from build123d import *

# Parameters (mm, degrees)
SKETCH_1_R      = 31.73899895
SKETCH_1_R_2    = 15.869499475
SKETCH_1_R_3    = 1.5
EXTRUDE_2_DEPTH = 2
EXTRUDE_3_DEPTH = 3
FILLET_1_R      = 1
FILLET_2_R      = 1
FILLET_3_R      = 1
FILLET_4_R      = 1
FILLET_5_R      = 1
FILLET_6_R      = 1
FILLET_7_R      = 1
FILLET_8_R      = 1


with BuildPart() as part:
    # 草图1 → 凸台-拉伸2 (new body)
    with BuildSketch(Plane.XY):
        Circle(SKETCH_1_R)
        Circle(SKETCH_1_R_2, mode=Mode.SUBTRACT)
        with Locations((-17, 17)):
            Circle(SKETCH_1_R_3, mode=Mode.SUBTRACT)
        with Locations((17, 17)):
            Circle(SKETCH_1_R_3, mode=Mode.SUBTRACT)
        with Locations((17, -17)):
            Circle(SKETCH_1_R_3, mode=Mode.SUBTRACT)
        with Locations((-17, -17)):
            Circle(SKETCH_1_R_3, mode=Mode.SUBTRACT)
        with Locations((-19.798989873, 19.798989873)):
            Circle(SKETCH_1_R_3, mode=Mode.SUBTRACT)
        with Locations((0, 28)):
            Circle(SKETCH_1_R_3, mode=Mode.SUBTRACT)
        with Locations((19.798989873, 19.798989873)):
            Circle(SKETCH_1_R_3, mode=Mode.SUBTRACT)
        with Locations((28, 0)):
            Circle(SKETCH_1_R_3, mode=Mode.SUBTRACT)
        with Locations((19.798989873, -19.798989873)):
            Circle(SKETCH_1_R_3, mode=Mode.SUBTRACT)
        with Locations((0, -28)):
            Circle(SKETCH_1_R_3, mode=Mode.SUBTRACT)
        with Locations((-19.798989873, -19.798989873)):
            Circle(SKETCH_1_R_3, mode=Mode.SUBTRACT)
        with Locations((-28, 0)):
            Circle(SKETCH_1_R_3, mode=Mode.SUBTRACT)
    extrude(amount=EXTRUDE_2_DEPTH)

    # 草图2 → 凸台-拉伸3 (add)
    with BuildSketch(Plane.XY.offset(2)):
        with BuildLine():
            Line((11.25, 23.25), (-11.25, 23.25))
            Line((-11.25, 23.25), (-11.25, 21.25))
            Line((-11.25, 21.25), (-4.584929155, 21.25))
            ThreePointArc((-4.584929155, 21.25), (0, 21.73899895), (4.584929155, 21.25))
            Line((4.584929155, 21.25), (11.25, 21.25))
            Line((11.25, 21.25), (11.25, 23.25))
        make_face()
        with BuildLine():
            Line((-23.25, 11.25), (-23.25, -11.25))
            Line((-23.25, -11.25), (-21.25, -11.25))
            Line((-21.25, -11.25), (-21.25, -4.584929155))
            ThreePointArc((-21.25, -4.584929155), (-21.73899895, 0), (-21.25, 4.584929155))
            Line((-21.25, 4.584929155), (-21.25, 11.25))
            Line((-21.25, 11.25), (-23.25, 11.25))
        make_face()
        with BuildLine():
            Line((21.25, -11.25), (23.25, -11.25))
            Line((23.25, -11.25), (23.25, 11.25))
            Line((23.25, 11.25), (21.25, 11.25))
            Line((21.25, 11.25), (21.25, 4.584929155))
            ThreePointArc((21.25, 4.584929155), (21.616403529, 2.305466077), (21.73899895, 0))
            ThreePointArc((21.73899895, 0), (21.616403529, -2.305466077), (21.25, -4.584929155))
            Line((21.25, -4.584929155), (21.25, -11.25))
        make_face()
        with BuildLine():
            Line((-11.25, -21.25), (-11.25, -23.25))
            Line((-11.25, -23.25), (11.25, -23.25))
            Line((11.25, -23.25), (11.25, -21.25))
            Line((11.25, -21.25), (4.584929155, -21.25))
            ThreePointArc((4.584929155, -21.25), (0, -21.73899895), (-4.584929155, -21.25))
            Line((-4.584929155, -21.25), (-11.25, -21.25))
        make_face()
        with BuildLine():
            ThreePointArc((-21.25, 4.584929155), (-21.73899895, 0), (-21.25, -4.584929155))
            Line((-21.25, -4.584929155), (-21.25, 4.584929155))
        make_face()
        with BuildLine():
            ThreePointArc((4.584929155, 21.25), (0, 21.73899895), (-4.584929155, 21.25))
            Line((-4.584929155, 21.25), (4.584929155, 21.25))
        make_face()
        with BuildLine():
            Line((21.25, 4.584929155), (21.25, -4.584929155))
            ThreePointArc((21.25, -4.584929155), (21.616403529, -2.305466077), (21.73899895, 0))
            ThreePointArc((21.73899895, 0), (21.616403529, 2.305466077), (21.25, 4.584929155))
        make_face()
    extrude(amount=EXTRUDE_3_DEPTH)

    # 圆角1
    fillet_1_edges = [part.edges().sort_by_distance(p)[0] for p in [
        (-22.25, -11.25, 5),
    ]]
    fillet(fillet_1_edges, radius=FILLET_1_R)

    # 圆角2
    fillet_2_edges = [part.edges().sort_by_distance(p)[0] for p in [
        (-22.25, 11.25, 5),
    ]]
    fillet(fillet_2_edges, radius=FILLET_2_R)

    # 圆角3
    fillet_3_edges = [part.edges().sort_by_distance(p)[0] for p in [
        (-11.25, 22.25, 5),
    ]]
    fillet(fillet_3_edges, radius=FILLET_3_R)

    # 圆角4
    fillet_4_edges = [part.edges().sort_by_distance(p)[0] for p in [
        (11.25, 22.25, 5),
    ]]
    fillet(fillet_4_edges, radius=FILLET_4_R)

    # 圆角5
    fillet_5_edges = [part.edges().sort_by_distance(p)[0] for p in [
        (22.25, 11.25, 5),
    ]]
    fillet(fillet_5_edges, radius=FILLET_5_R)

    # 圆角6
    fillet_6_edges = [part.edges().sort_by_distance(p)[0] for p in [
        (22.25, -11.25, 5),
    ]]
    fillet(fillet_6_edges, radius=FILLET_6_R)

    # 圆角7
    fillet_7_edges = [part.edges().sort_by_distance(p)[0] for p in [
        (11.25, -22.25, 5),
    ]]
    fillet(fillet_7_edges, radius=FILLET_7_R)

    # 圆角8
    fillet_8_edges = [part.edges().sort_by_distance(p)[0] for p in [
        (-11.25, -22.25, 5),
    ]]
    fillet(fillet_8_edges, radius=FILLET_8_R)


solid = part.part
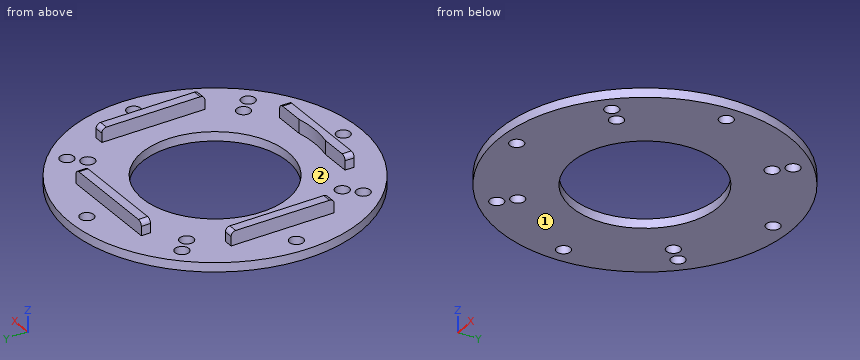
Can you work these out from the model? Positions are in its coordinate system, mm. Face numbers are marked on the shaded views. Coordinates: 2 decimals unless noted, no trailing zeros. Write each loop counter-clockwise with the first axis right and the second up, starting at its lowest first coordinate (ties: lowest second). Pieces come first, ordered by that corner, then holes. Notation, with made-up numbers: (5, -5) - (36, -5) arc R18 ccw to (36, 14) - close; hole circle Ø10 at (-27.5, -6). An arc over 180 degrees is marked (long way). Return JSON: item names as keys, results as strings. Group by question number.
Item 1: If we section it at C-C (x = -20): Write out the boundary of the cut face in (y, z).
Item 2: If we section it at D-D (x = -28): Write out the boundary of the cut face in (y, z), then the cut area to 3 significant figures.
Item 3: Please list where these lines run through material, in increasing order: probe 1 along Y at (x, z) = (-8, 2.85); probe 2 along Y at (x, z) = (20.5, 0.4); probe 3 along Y at (x, z) = (17, 0.95).
Item 4: If we section it at B-B (y = 0): Write out the boundary of the cut face in (x, z), then the cut area to 3 significant figures.
Item 5: I'm going to push flat-ended pins straight in: pin 1 Ø1.5 at (x, y) = (4.5, -16) entering from +Z; pin 2 Ø1.5 at (x, y) = (-18.5, -20.5) entering from -Z; pin 3 Ø1 at (x, z) = (-21, 4.5) entering from +Y; pin 4 Ø1.5 at (y, z) = (1.5, 3.5) entering from -X. Where does each tip first touch, or does it pass through?
Item 6: If we section it at A-A (x = 0): Write out the boundary of the cut face in (y, z).
Item 7: We'd pull the mould along Y, two halves only. Please class the marked faces 1 and 2: pulls with the +Y half, pulls with the -Y half, needs draft (parallel to the pull), parting line crosses it, or undercut.
Return value:
{
 "1": {"outline": "(-24.64, 0) - (-21.29, 0) - (-21.29, 2) - (-24.64, 2) - close; (-18.31, 0) - (18.31, 0) - (18.31, 2) - (-18.31, 2) - close; (21.29, 0) - (24.64, 0) - (24.64, 2) - (21.29, 2) - close"},
 "2": {"outline": "(-14.95, 0) - (-1.5, 0) - (-1.5, 2) - (-14.95, 2) - close; (1.5, 0) - (14.95, 0) - (14.95, 2) - (1.5, 2) - close", "area": "53.8 mm^2"},
 "3": {"probe 1": "y = -23.25 to -21.25, 21.25 to 23.25", "probe 2": "y = -24.23 to -21.13, -18.47 to 18.47, 21.13 to 24.23", "probe 3": "y = -26.8 to -18.5, -15.5 to 15.5, 18.5 to 26.8"},
 "4": {"outline": "(-31.74, 0) - (-29.5, 0) - (-29.5, 2) - (-31.74, 2) - close; (-26.5, 0) - (-15.87, 0) - (-15.87, 2) - (-21.25, 2) - (-21.25, 5) - (-23.25, 5) - (-23.25, 2) - (-26.5, 2) - close; (15.87, 0) - (26.5, 0) - (26.5, 2) - (23.25, 2) - (23.25, 5) - (21.25, 5) - (21.25, 2) - (15.87, 2) - close; (29.5, 0) - (31.74, 0) - (31.74, 2) - (29.5, 2) - close", "area": "63.5 mm^2"},
 "5": {"pin 1": "stops at z = 2", "pin 2": "stops at z = 0", "pin 3": "stops at y = 11.25", "pin 4": "stops at x = -23.25"},
 "6": {"outline": "(-31.74, 0) - (-29.5, 0) - (-29.5, 2) - (-31.74, 2) - close; (-26.5, 0) - (-15.87, 0) - (-15.87, 2) - (-21.74, 2) - (-21.74, 5) - (-23.25, 5) - (-23.25, 2) - (-26.5, 2) - close; (15.87, 0) - (26.5, 0) - (26.5, 2) - (23.25, 2) - (23.25, 5) - (21.25, 5) - (21.25, 2) - (15.87, 2) - close; (29.5, 0) - (31.74, 0) - (31.74, 2) - (29.5, 2) - close"},
 "7": {"face 1": "needs draft", "face 2": "undercut"}
}
